Autodesk Inventor part; units mm, degrees
sketch "スケッチ1" plane through (0, 0, 0) normal (0, 0, 1) x (1, 0, 0)
  circle A0 centre (0, 0) radius 10.85
  dimension "d0" = 21.7
extrude "押し出し1" add sketch "スケッチ1" along normal blind 1.95
sketch "スケッチ2" plane through (0, 0, 0) normal (0, 0, 1) x (1, 0, 0)
  circle A0 centre (0, 0) radius 4.7
  dimension "d3" = 9.4
extrude "押し出し2" add sketch "スケッチ2" against normal blind 3.5
sketch "スケッチ3" plane through (0, 0, 0) normal (0, 0, 1) x (1, 0, 0)
  circle A0 centre (0, 0) radius 3
  dimension "d6" = 6
extrude "押し出し3" cut sketch "スケッチ3" against normal blind 3.5
sketch "スケッチ4" plane through (0, 0, 0) normal (0, 0, 1) x (1, 0, 0)
  circle A0 centre (0, 0) radius 4.2
  dimension "d9" = 8.4
extrude "押し出し4" add sketch "スケッチ4" along normal blind 2.5
sketch "スケッチ5" plane through (0, 0, 2.5) normal (0, 0, 1) x (1, 0, 0)
  circle A0 centre (0, 0) radius 3.5
  dimension "d12" = 7
extrude "押し出し5" cut sketch "スケッチ5" against normal blind 1.4
sketch "スケッチ6" plane through (0, 0, 0) normal (0, 0, 1) x (1, 0, 0)
  circle A0 centre (0, 0) radius 1.7
  dimension "d15" = 3.4
extrude "押し出し6" cut sketch "スケッチ6" along normal through all
sketch "スケッチ7" plane through (0, 0, 0) normal (0, 0, 1) x (1, 0, 0)
  circle A0 centre (7.8, 0) radius 0.8
  point P0 (0, 0)
  dimension "d18" = 1.6
  dimension "d19" = 7.8
extrude "押し出し7" cut sketch "スケッチ7" along normal through all
pattern_circular "円形状パターン1" count 4 over 360 about axis through (0, 0, -10) along (0, 0, 1) of "押し出し7"
chamfer "面取り1" distance 0.2 angle 45 1 edges at (-4.7, 0, 0)
properties part number "HbServoHorn01"
Input: part model. Units: mm. Frame: model coordinates. A direction names the side the tool comes from. Round coordinates to 2 decimals unless told otherwise and drop trailing zeros. Loops run counter-clockwise (first coordinate to the right, second up) from the corner with the lowest first, then second, coordinate; pieces in that order, holes last. Notation, with made-up numbers: (55, 48.25) - (60, 48.25) arc R18 cw to (60, 61.25) - close; hole circle Ø6 at (16, 22.25). An arc over 180 degrees is marked (long way). One line per item, written item: value. Start each with the question number.
(1) Draft query along Y for faces 1 (the cylindrical face through (-1.02, -4.59, -1.83)), 2 (the flat face through (5, -2, 0)), 3 (the cylindrical face through (-0.37, 1.66, 0.54)). Return one class per face: +Y half, -Y half, draft (parallel to the pull), parting line (faces both ways), or undercut.
(2) Section A-A, the plane y = -7.5. Return loops of the section in (x, z).
(3) Section B-B, the plane x = 0. Count the separate pieces of the cut face and the enclosed holes in it, plus the area to 3 significant figures.
(4) Section D-D, the plane z = -2.7. Return loops of the section in (x, y), plus the area to 3 significant figures.
(5) Contact query for flat-ended pins moving along their axis: P1, Ø1, axis at x = 2, y = 6.5, coming from the -Z side; P2, Ø5.5, axis at x = -0.5, y = -0.5, coming from the +Z side; P3, Ø3, axis at x = 0, y = 0, coming from the -Z side; P4, Ø1.8, axis at x = 0, y = 7.8, coming from the +Z side. Output: stop coordinate, or through.
(6) Access query for faces 4 (the cylindrical face through (-0.306, 8.539, 0.961)), 5 (the cylindrical face through (3.233, -1.341, 1.81)), 6 (the cylindrical face through (-3, 0, -2)). Directions: +Z, -Z, +X, -X, +Y, -Y. A direction counts if a zero-diameter tool reaches every point of the face in a straight line with its end or side. Return the directions, or none.
(7) Ray query, line 1 (Y direction, x = 0, z = 1.05); line 2 (Y direction, x = 0, z = 1.3); line 3 (Z direction, x = 7.25, y = -5.5). Return the intervals inside material, ascending. Write a range as [from, to].
Results below:
1. face 1: parting line
1. face 2: draft
1. face 3: undercut
2. outline: (-7.84, 0) - (-0.74, 0) - (-0.74, 1.95) - (-7.84, 1.95) - close; (0.74, 0) - (7.84, 0) - (7.84, 1.95) - (0.74, 1.95) - close
3. separate pieces: 4
3. enclosed holes: 0
3. area: 39.1 mm^2
4. outline: circle Ø9.4 at (0, 0); hole circle Ø6 at (0, 0)
4. area: 41.1 mm^2
5. P1: z = 0
5. P2: z = 1.1
5. P3: through
5. P4: z = 1.95
6. face 4: +Z, -Z
6. face 5: +Z
6. face 6: -Z
7. line 1: [-10.85, -8.6], [-7, -1.7], [1.7, 7], [8.6, 10.85]
7. line 2: [-10.85, -8.6], [-7, -3.5], [3.5, 7], [8.6, 10.85]
7. line 3: [0, 1.95]
